Input: dimensioned drawing with shaded views. Units: mm. Origin: part minimum x, y, z. Round coordinates to 2 decimals unless told otherwise and drop trailing zeros. Write each loop counter-clockwise with the first axis right and the second up, starting at its lowest first coordinate (ties: lowest second). Pieces come first, ordered by that corner, then holes. Notation, with made-up numbers: (77.5, -34.5) -> (93.5, -34.5) arc R9 cw to (93.5, -27.5) -> close; hole circle Ø10 at (-38.5, 26). An arc over 180 degrees is marked (long way). Use one line per item in the form item = value. Start each with the question number.
1. Cut plane B-B, the plane z = 14.25. Return the cut outline in (x, y).
2. Cut plane A-A, the plane x = 35.25. Return the cut outline in (y, z).
3. Cut plane C-C, the plane z = 22. Return the cut outline in (x, y).
4. Line query: L1, parallel to Y at x = 6, z = 9.5; L2, parallel to Y at x = 39, z = 7.75. Output: solid intervals per line, ascending.
5. Cut plane D-D, the plane x = 13. Return the cut outline in (y, z).
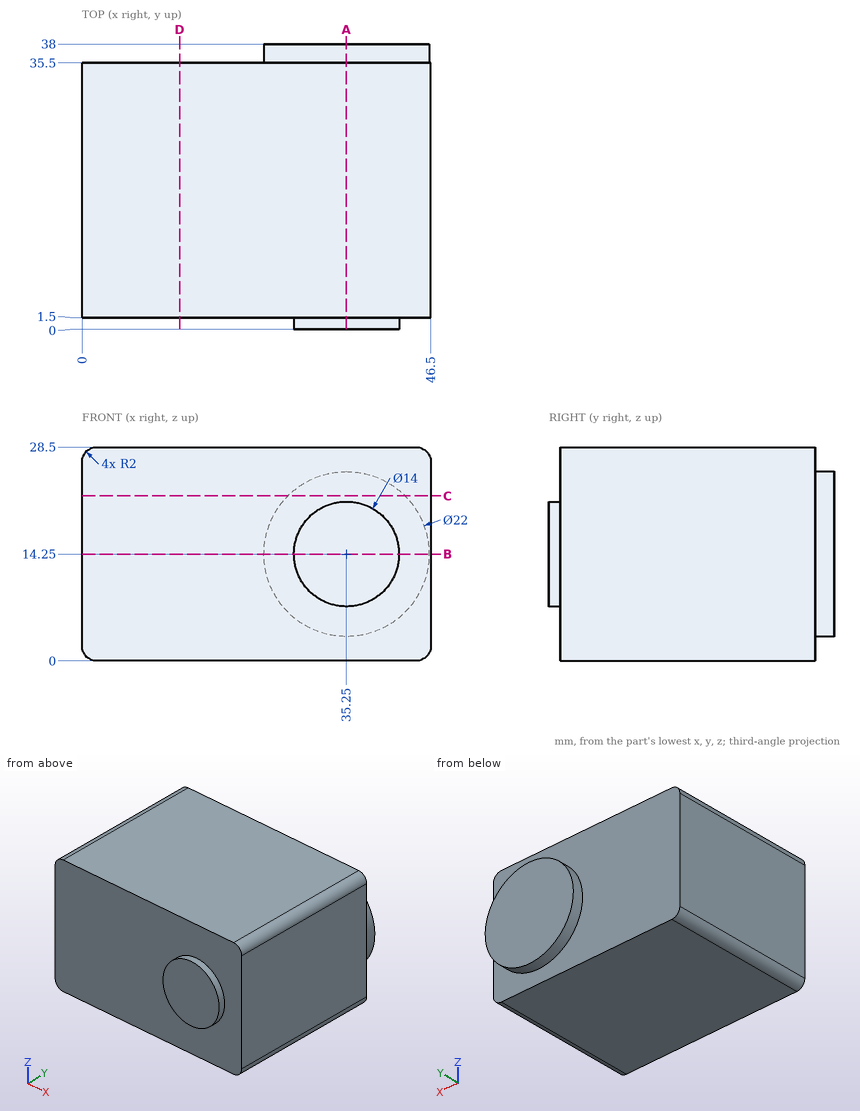
Outcome:
q1.outline = (0, 1.5) -> (28.25, 1.5) -> (28.25, 0) -> (42.25, 0) -> (42.25, 1.5) -> (46.5, 1.5) -> (46.5, 35.5) -> (46.25, 35.5) -> (46.25, 38) -> (24.25, 38) -> (24.25, 35.5) -> (0, 35.5) -> close
q2.outline = (0, 7.25) -> (1.5, 7.25) -> (1.5, 0) -> (35.5, 0) -> (35.5, 3.25) -> (38, 3.25) -> (38, 25.25) -> (35.5, 25.25) -> (35.5, 28.5) -> (1.5, 28.5) -> (1.5, 21.25) -> (0, 21.25) -> close
q3.outline = (0, 1.5) -> (46.5, 1.5) -> (46.5, 35.5) -> (43.06, 35.5) -> (43.06, 38) -> (27.44, 38) -> (27.44, 35.5) -> (0, 35.5) -> close
q4.L1 = 1.5 to 35.5
q4.L2 = 1.5 to 38
q5.outline = (1.5, 0) -> (35.5, 0) -> (35.5, 28.5) -> (1.5, 28.5) -> close
